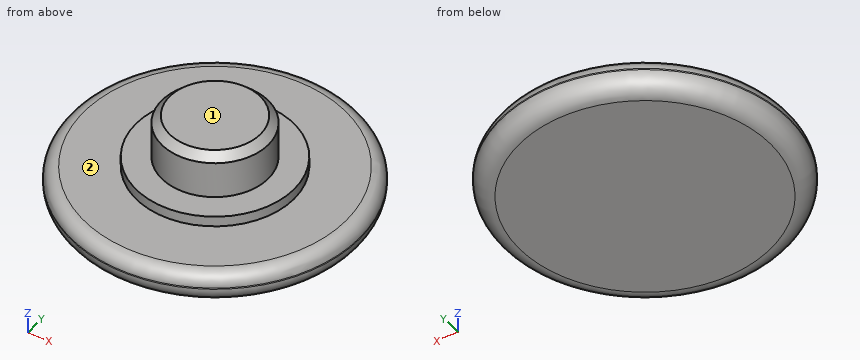
```python
from build123d import *

# Parameters (mm, degrees)
F0_R     = 10.95
F1_DEPTH = 2.5
F2_R     = 4.05
F3_DEPTH = 4.2
F4_R     = 1
F5_R     = 6
F6_DEPTH = 0.8
F7_R     = 1.4
F8_SIZE  = 0.6


with BuildPart() as f1:
    # F0 (on Top) → F1 (new body)
    with BuildSketch(Plane.XY):
        Circle(F0_R)
    extrude(amount=F1_DEPTH)

    # F2 (on face) → F3 (join)
    with BuildSketch(Plane.XY.offset(2.5)):
        Circle(F2_R)
    extrude(amount=F3_DEPTH)

    # F4
    f4_edges = [f1.edges().sort_by_distance(p)[0] for p in [
        (-10.95, 0, 2.5),
    ]]
    fillet(f4_edges, radius=F4_R)

    # F5 (on face) → F6 (join)
    with BuildSketch(Plane.XY.offset(2.5)):
        Circle(F5_R)
    extrude(amount=F6_DEPTH)

    # F7
    f7_edges = [f1.edges().sort_by_distance(p)[0] for p in [
        (-10.95, 0, 0),
    ]]
    fillet(f7_edges, radius=F7_R)

    # F8
    f8_edges = [f1.edges().sort_by_distance(p)[0] for p in [
        (-4.05, 0, 6.7),
    ]]
    chamfer(f8_edges, length=F8_SIZE)


solid = f1.part
```
Geometry check sheet. Reference: the model listing, model coordinates, mm. Face numbers are marked on the shaded views. A direction names the side the tool comes from. Give positions to 0.01 mm unless a question says otherwise; leave off trailing zeros. Order: outer loops, then holes, each group sorted by start corner. A loop starts at its lowest first (then second) coordinate and runs counter-clockwise, first axis right, second up. Notation, with made-up numbers: (58.25, 10) -> (62.25, 10) arc R19 cw to (62.25, 26) -> close; hole circle Ø7 at (16.25, -32.5). An arc over 180 degrees is marked (long way). Write each question's results on one line, items separated by ' | '. Start each with the question number.
(1) Gauge pin test, flat ends, axial feed: P1, Ø8, axis at x = -4, y = -6.5, coming from the +Z side; P2, Ø1, axis at x = 1, z = 3.5, coming from the +Y side; P3, Ø1, axis at x = 6.5, y = -4.5, coming from the +Z side; P4, Ø1.5, axis at x = -7, y = -0.5, coming from the -Z side. Record the tip position at first contact, or that the pin passes through.
(2) Access from +Z, -Z, +X, -X, +Y, -Y to the whole of each face (thin tool, end or side, straight path). Record for the marked faces 1 and 2.
(3) Scan lines: line 1 (Z direction, x = -6, y = -5.75); line 2 (Z direction, x = -3.5, y = -4.25); line 3 (X direction, y = -0.25, z = 1.5). Record each from-to range of solid material in increasing order.
(4) Sectioned sample at D-D (z = 3). Enter the section's corners in (x, y), plus the area to 3 significant figures.
(5) Sectioned sample at C-C (z = 4.25). Enter the section's corners in (x, y), plus the area to 3 significant figures.
(6) Sectioned sample at A-A (y = 0). Enter the section's corners in (x, z).
Answer below:
1) P1: z = 6.52 | P2: y = 5.98 | P3: z = 2.5 | P4: z = 0
2) face 1: +Z, +X, -X, +Y, -Y | face 2: +Z
3) line 1: 0 to 2.5 | line 2: 0 to 3.3 | line 3: -10.95 to 10.95
4) outline: circle Ø12 at (0, 0) | area: 113 mm2
5) outline: circle Ø8.1 at (0, 0) | area: 51.5 mm2
6) outline: (-10.95, 1.4) arc R1.4 ccw to (-9.55, 0) -> (9.55, 0) arc R1.4 ccw to (10.95, 1.4) -> (10.95, 1.5) arc R1 ccw to (9.95, 2.5) -> (6, 2.5) -> (6, 3.3) -> (4.05, 3.3) -> (4.05, 6.1) -> (3.45, 6.7) -> (-3.45, 6.7) -> (-4.05, 6.1) -> (-4.05, 3.3) -> (-6, 3.3) -> (-6, 2.5) -> (-9.95, 2.5) arc R1 ccw to (-10.95, 1.5) -> close
